Could you check a few things on this model? Use its own coordinates, in mm. A direction names the side the tool comes from. Round coordinates to 2 decimals unless told otherwise and drop trailing zeros. Loops run counter-clockwise (first coordinate to the right, second up) from the corner with the lowest first, then second, coordinate; pieces in that order, holes last. Notation, with made-up numbers: (-22.75, 3.5) - (10.25, 3.5) arc R21 cw to (10.25, 29.5) - close; hole circle Ø1 at (79, -0.5). An arc over 180 degrees is marked (long way). Use one line per item in the form item = value.
```python
from build123d import *

# Parameters (mm, degrees)
F0_W     = 115
F0_H     = 85
F1_DEPTH = 2
F2_W     = 115
F2_H     = 85
F2_W_2   = 112
F2_H_2   = 82
F3_DEPTH = 4
F4_W     = 115
F4_H     = 85
F5_DEPTH = 1.5
F6_W     = 82
F6_H     = 4.5
F7_DEPTH = 7.1
F8_W     = 96.06551
F8_H     = 30.124249
F8_H_2   = 30.12425
F9_DEPTH = 20


with BuildPart() as f1:
    # F0 (on Top) → F1 (new body)
    with BuildSketch(Plane.XY):
        with Locations((17.203308, 3.536641)):
            Rectangle(F0_W, F0_H)
    extrude(amount=F1_DEPTH)

    # F2 (on face) → F3 (join)
    with BuildSketch(Plane.XY.offset(2)):
        with Locations((17.203308, 3.536641)):
            Rectangle(F2_W, F2_H)
        with Locations((17.203308, 3.536641)):
            Rectangle(F2_W_2, F2_H_2, mode=Mode.SUBTRACT)
    extrude(amount=F3_DEPTH)

    # F4 (on face) → F5 (join)
    with BuildSketch(Plane.XY.offset(6)):
        with Locations((17.203308, 3.536641)):
            Rectangle(F4_W, F4_H)
    extrude(amount=F5_DEPTH)

    # F6 (on face) → F7 (cut)
    with BuildSketch(Plane.YZ.offset(74.703308)):
        with Locations((3.536641, 3.75)):
            Rectangle(F6_W, F6_H)
    extrude(amount=-F7_DEPTH, mode=Mode.SUBTRACT)

    # F8 (on face) → F9 (cut)
    with BuildSketch(Plane.XY.offset(7.5)):
        with Locations((16.722513, 22.296688)):
            Rectangle(F8_W, F8_H)
        with Locations((16.722513, -15.223406)):
            Rectangle(F8_W, F8_H_2)
    extrude(amount=-F9_DEPTH, mode=Mode.SUBTRACT)


solid = f1.part
```
1. Please list where these lines run through material, in increasing order: line 1 along Y through (x, z) = (16.5, 6.25); line 2 along Y through (x, z) = (-30, 4.5); line 3 along Z through (x, y) = (4, 0).
Solution:
line_1 = -38.96 to -30.29, -0.16 to 7.23, 37.36 to 46.04
line_2 = -38.96 to -37.46, 44.54 to 46.04
line_3 = 0 to 2, 6 to 7.5
2. We'd pull the mould along Y, two halves only. Please class faces 3 (the face through (19, 44.537, 4)), 4 (the face through (-40.297, 3, 4)), 5 (the face through (16, 46.037, 4)): +Y half, -Y half, draft (parallel to the pull), parting line (faces both ways), or undercut.
Solution:
face_3 = undercut
face_4 = draft
face_5 = +Y half
3. For P1, Ø0.6, axis at y = 23, z = 2, coming from the +X side, with a flat end and sliding along its axis, tell me the tip position at first contact or that it passes through.
Solution:
P1 = 67.6
4. If we section it at A-A, the plane y = 22.5: Write out the boundary of the cut face in (x, z), plus the area to 3 significant figures.
Solution:
outline = (-40.3, 0) - (-31.31, 0) - (-31.31, 2) - (-38.8, 2) - (-38.8, 6) - (-31.31, 6) - (-31.31, 7.5) - (-40.3, 7.5) - close; (64.76, 0) - (74.7, 0) - (74.7, 1.5) - (67.6, 1.5) - (67.6, 2) - (64.76, 2) - close; (64.76, 6) - (74.7, 6) - (74.7, 7.5) - (64.76, 7.5) - close
area = 68.7 mm^2
5. If we section it at D-D, the plane z = 4: Write out the boundary of the cut face in (x, y), plus the area to 3 significant figures.
Solution:
outline = (-40.3, -38.96) - (74.7, -38.96) - (74.7, -37.46) - (-38.8, -37.46) - (-38.8, 44.54) - (74.7, 44.54) - (74.7, 46.04) - (-40.3, 46.04) - close
area = 468 mm^2
6. If we section it at B-B, the plane x = 37.5: Write out the boundary of the cut face in (y, z).
Solution:
outline = (-38.96, 0) - (-30.29, 0) - (-30.29, 2) - (-37.46, 2) - (-37.46, 6) - (-30.29, 6) - (-30.29, 7.5) - (-38.96, 7.5) - close; (-0.16, 0) - (7.23, 0) - (7.23, 2) - (-0.16, 2) - close; (-0.16, 6) - (7.23, 6) - (7.23, 7.5) - (-0.16, 7.5) - close; (37.36, 0) - (46.04, 0) - (46.04, 7.5) - (37.36, 7.5) - (37.36, 6) - (44.54, 6) - (44.54, 2) - (37.36, 2) - close
7. On a 3-axis mill with a long thin cutter (end or side, diameter ignored), from which of +Z, -Z, +X, -X, +Y, -Y can I reach the whole of each face in a straight line? I mean faces 1 (the face through (16, 4, 7.5)), 2 (the face through (-38.797, 3, 4)). Say none if no direction works.
Solution:
face_1 = +Z, +X, -X, +Y, -Y
face_2 = +X
8. If we section it at C-C, the plane y = 4: Write out the boundary of the cut face in (x, z).
Solution:
outline = (-40.3, 0) - (74.7, 0) - (74.7, 1.5) - (67.6, 1.5) - (67.6, 2) - (-38.8, 2) - (-38.8, 6) - (74.7, 6) - (74.7, 7.5) - (-40.3, 7.5) - close
